The figure shows three views and two pictorial views of one solid part (mm, origin at its lowest corner). Answer the questions. Round coordinates to 2 decimals unless told otherwise and drop trailing zeros. Order: outer loops, then holes, each group sorted by start corner. A loop starts at its lowest first (then second) coordinate and runs counter-clockwise, first axis right, second up. Notation, with made-up numbers: M 12,34.25 L 38,34.25 A15 cw 38,61.25 Z; hole C 32,-20.5 d2. An arc over 180 degrees is marked long. Return JSON: item names as keys, results as strings.
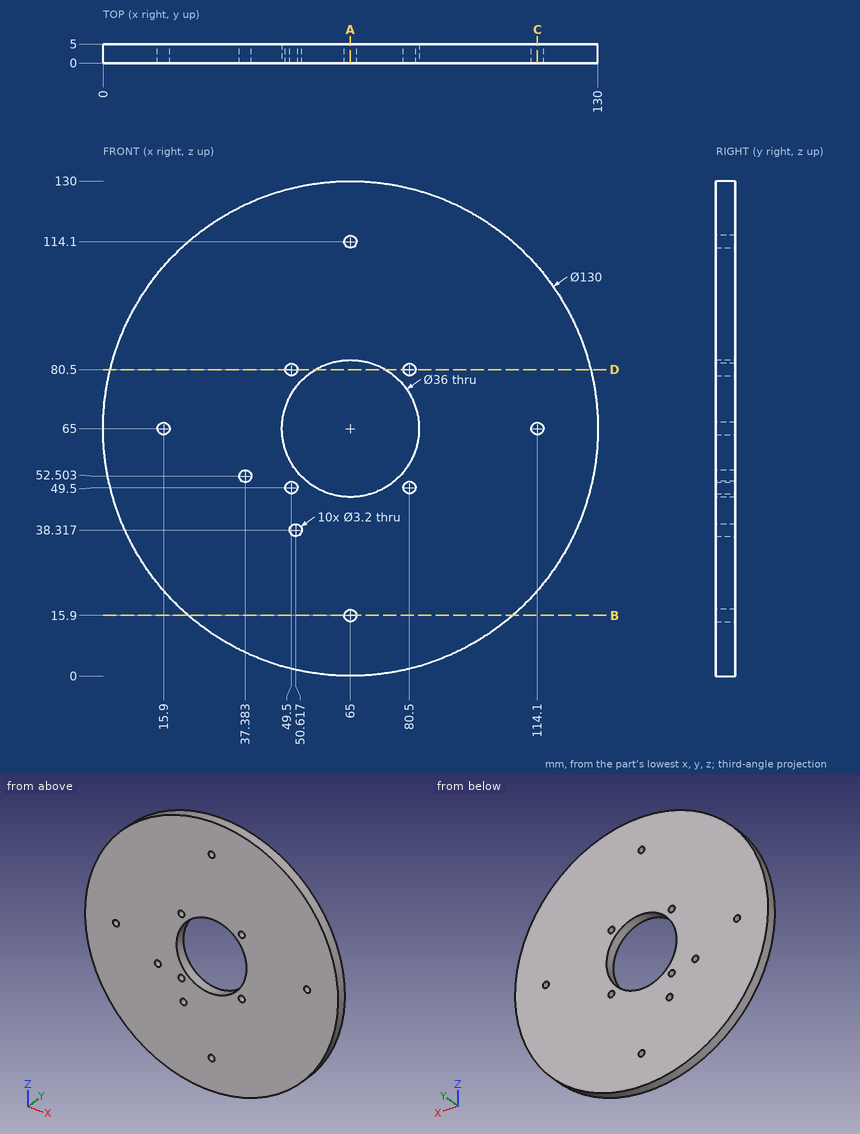
Item 1: Consider line 1 along X through (y, z) = (3.45, 65); line 2 along X through (y, z) = (1.2, 56.5); line 3 along X through (y, z) = (4.2, 68). Determine where each line is inside the solid, lowest interval first. Write a range as [from, to].
Output:
{"line 1": "x = [0, 14.3], [17.5, 47], [83, 112.5], [115.7, 130]", "line 2": "x = [0.56, 49.13], [80.87, 129.44]", "line 3": "x = [0.07, 47.25], [82.75, 129.93]"}
Item 2: Find section B-B (z = 15.9). Determine the outline of the cut face in (x, y).
Output:
{"outline": "M 22.41,0 L 63.4,0 L 63.4,5 L 22.41,5 Z; M 66.6,0 L 107.59,0 L 107.59,5 L 66.6,5 Z"}
Item 3: Each of these flat-tipped pins is pushed along its axis until it touches: pin 1 (3 mm diameter, centred on x = 65, z = 15.9, fed in from -Y); pin 2 (1.5 mm diameter, centred on y = 2, z = 67, fed in from +X). Where does it stop, or does it pass through?
Output:
{"pin 1": "passes through", "pin 2": "stops at x = 129.99"}
Item 4: Find section C-C (x = 114.1). Determine the outline of the cut face in (y, z), plus the area to 3 significant figures.
Output:
{"outline": "M 0,22.41 L 5,22.41 L 5,63.4 L 0,63.4 Z; M 0,66.6 L 5,66.6 L 5,107.59 L 0,107.59 Z", "area": "410 mm^2"}
Item 5: Find section D-D (z = 80.5). Determine the outline of the cut face in (x, y) (1 decimal).
Output:
{"outline": "M 1.9,0 L 47.9,0 L 47.9,5 L 1.9,5 Z; M 51.1,0 L 55.8,0 L 55.8,5 L 51.1,5 Z; M 74.2,0 L 78.9,0 L 78.9,5 L 74.2,5 Z; M 82.1,0 L 128.1,0 L 128.1,5 L 82.1,5 Z"}
Item 6: Find section A-A (x = 65). Determine the outline of the cut face in (y, z), plus the area to 3 significant figures.
Output:
{"outline": "M 0,0 L 5,0 L 5,14.3 L 0,14.3 Z; M 0,17.5 L 5,17.5 L 5,47 L 0,47 Z; M 0,83 L 5,83 L 5,112.5 L 0,112.5 Z; M 0,115.7 L 5,115.7 L 5,130 L 0,130 Z", "area": "438 mm^2"}
